Verification items for the finished model (mm, model axes). A direction names the side the tool comes from. Coordinates: 2 decimals unless noted, no trailing zeros. Order: outer loops, then holes, each group sorted by start corner. A loop starts at its lowest first (then second) coordinate and runs counter-clockwise, first axis right, second up. Notation, with made-up numbers: (66, 42) -> (88, 42) arc R24 ccw to (88, 80) -> close; hole circle Ø8 at (27.5, 25.5). An arc over 180 degrees is marked (long way). Write each question's results on one line, items separated by ' | '. Start each with the question number.
(1) Cross-section at A-A on z = 4. Enter the section's corners in (x, y) (3 decimals), and give its area (3 significant figures).
(2) Draft check along X on faces 1 (the flat face through (1, -36, 9.525)), 2 (the cylindrical face through (32.73, -16.79, 51.97)), 3 (the flat face through (60.325, 0, 41)). Enter one of: +X half, -X half, draft (parallel to the pull), parting line (faces both ways), or undercut.
(3) Go/stop test with flat-tipped pins: pin 1 (5 mm diameter, centred on y = -13, z = 14.5, fed in from -X) (3 decimals); pin 2 (2.5 mm diameter, centred on x = 59, y = -18, fed in from +Z); pin 3 (5 mm diameter, centred on x = 18, z = 52.5, fed in from -Y). Record where each tip stops, or that it passes through.
(4) Thickness scan on probe 1 along Z at (x, y) = (10.5, -36.5) (3 decimals); probe 2 along Z at (x, y) = (103, 14.5) (3 decimals); probe 3 along Y at (x, z) = (4.5, 49). Record the ranges inside material, lowest first. Write a range as [from, to].
(5) Cross-section at D-D on y = -13.5. Enter the section's corners in (x, z) (3 decimals).
(6) Set-up check for faces 4 (the flat face through (-1, 7.938, 32)), 5 (the flat face through (41.275, -1, 4)), 6 (the flat face through (22.225, -17, 18)): record each of +Z, -Z, +X, -X, +Y, -Y from which the full face is reachable in a straight line by a thin tool's end or side.
(7) Cross-section at B-B on y = 38.5. Enter the section's corners in (x, z) (3 decimals), and give its area (3 significant figures).
(8) Cross-section at C-C on x = 71.5. Enter the section's corners in (y, z) (3 decimals).
```python
from build123d import *

# Parameters (mm, degrees)
F1_DEPTH = 63.5
F2_DEPTH = 25.4
F3_DEPTH = 7.9375
F0_W     = 25.4
F0_H     = 28.575
F5_R     = 6.35


with BuildPart() as f1:
    # F0 (on Front) → F1 (new body, symmetric)
    with BuildSketch(Plane.XZ):
        Polygon((-41.275, 9.525), (-41.275, -9.525), (41.275, -9.525), (41.275, 9.525), (22.225, 9.525), align=None)
    extrude(amount=F1_DEPTH, both=True)

    # F0 (on Front) → F2 (join, symmetric)
    with BuildSketch(Plane.XZ):
        with BuildLine():
            Line((22.225, 9.525), (41.275, 9.525))
            Line((41.275, 9.525), (41.275, 27.0002))
            ThreePointArc((41.275, 27.0002), (45.92468, 38.22552), (57.15, 42.8752))
            Line((57.15, 42.8752), (60.325, 42.8752))
            Line((60.325, 42.8752), (60.325, 61.9252))
            Line((60.325, 61.9252), (57.15, 61.9252))
            ThreePointArc((57.15, 61.9252), (32.454296, 51.695904), (22.225, 27.0002))
            Line((22.225, 27.0002), (22.225, 9.525))
        make_face()
        Polygon((60.325, 66.675), (60.325, 61.9252), (60.325, 42.8752), (60.325, 38.1), (85.725, 38.1), (85.725, 66.675), align=None)
    extrude(amount=F2_DEPTH, both=True)

    # F0 (on Front) → F3 (join, symmetric)
    with BuildSketch(Plane.XZ):
        with BuildLine():
            add(Edge.make_bspline(
                [(-41.275, 9.525), (-27.082177, 48.334144), (26.706019, 66.012785), (60.325, 61.9252)],
                knots=[0, 0, 0, 0, 114.316845, 114.316845, 114.316845, 114.316845], degree=3))
            Line((-41.275, 9.525), (22.225, 9.525))
            Line((22.225, 9.525), (22.225, 27.0002))
            ThreePointArc((22.225, 27.0002), (32.454296, 51.695904), (57.15, 61.9252))
            Line((57.15, 61.9252), (60.325, 61.9252))
        make_face()
    extrude(amount=F3_DEPTH, both=True)

    # F0 (on Front) → F4 (revolve)
    with BuildSketch(Plane.XZ):
        with Locations((98.425, 52.3875)):
            Rectangle(F0_W, F0_H)
    revolve(axis=Axis((85.725, 0, 52.3875), (0, 0, 1)))

    # F5
    f5_edges = [f1.edges().sort_by_distance(p)[0] for p in [
        (-41.275, -63.5, 0),
        (41.275, -63.5, 0),
        (41.275, 63.5, 0),
        (-41.275, 63.5, 0),
    ]]
    fillet(f5_edges, radius=F5_R)


solid = f1.part
```
Results are:
1) outline: (-41.275, -57.15) arc R6.35 ccw to (-34.925, -63.5) -> (34.925, -63.5) arc R6.35 ccw to (41.275, -57.15) -> (41.275, 57.15) arc R6.35 ccw to (34.925, 63.5) -> (-34.925, 63.5) arc R6.35 ccw to (-41.275, 57.15) -> close | area: 10,400 mm2
2) face 1: draft | face 2: -X half | face 3: undercut
3) pin 1: stops at x = 22.225 | pin 2: stops at z = 61.93 | pin 3: stops at y = -7.94
4) probe 1: z = [-9.525, 9.525] | probe 2: z = [38.1, 66.675] | probe 3: y = [-7.94, 7.94]
5) outline: (-41.275, -9.525) -> (41.275, -9.525) -> (41.275, 27) arc R15.875 cw to (57.15, 42.875) -> (60.325, 42.875) -> (60.325, 38.1) -> (107.24, 38.1) -> (107.24, 66.675) -> (60.325, 66.675) -> (60.325, 61.925) -> (57.15, 61.925) arc R34.925 ccw to (22.225, 27) -> (22.225, 9.525) -> (-41.275, 9.525) -> close
6) face 4: +Z, -X, +Y | face 5: -Z, +X, +Y, -Y | face 6: +Z, -X, -Y
7) outline: (-41.275, -9.525) -> (41.275, -9.525) -> (41.275, 9.525) -> (-41.275, 9.525) -> close | area: 1,570 mm2
8) outline: (-25.4, 38.1) -> (25.4, 38.1) -> (25.4, 66.675) -> (-25.4, 66.675) -> close
